For this review, take the finished solid that the model builds, in its own axes (mm). A direction names the side the tool comes from. Coordinates: 2 decimals unless noted, no trailing zeros. Loops run counter-clockwise (first coordinate to the right, second up) from the corner with the lowest first, then second, coordinate; pieces in that order, holes last. Notation, with made-up numbers: (-5.75, -34) - (45.25, -34) arc R6 cw to (45.25, -24) - close; hole circle Ø3 at (3, 54). An arc over 180 degrees is marked (long way). Answer as a JSON object with one key per item and string values. Group by question number.
Item 1: We need section A-A (y = 17.5). Give the boundary of the cut face in (x, z).
Item 2: Mouldability with a two-part tool opening along X and no side actions: class faces 4 (the flat face through (21, 2, -17)), 5 (the flat face through (0, 19, 4.3)) as released by +X, released by -X, zero draft, split by the parting line, or undercut.
Item 3: Clearance check with flat-ended pins moving along their axes: pin 1 (1.1 mm diameter, centred on x = 44, z = -35, fed in from +Y); pin 2 (1 mm diameter, centred on x = 33.5, y = 13, fed in from +Z); pin 3 (2 mm diameter, centred on x = -1.5, y = 7.5, fed in from -Z); pin 4 (4 mm diameter, centred on y = 13.5, z = -22, fed in from -X). State where each tip first meets the part, or that it passes through.
Item 4: We need section B-B (y = 9). Give the boundary of the cut face in (x, z), then the cut area to 3 significant figures.
Item 5: Tool access review of faces 1 (the flat face through (42.3, 19, 3)), 2 (the flat face through (45, 19, -15.2)), 3 (the flat face through (44.3, 10, -20)): name each direction out of +Z, -Z, +X, -X, +Y, -Y from which nothing blocks a thin tool from reaching the whole face with its end or side.
Item 6: To check wall thickness, follow line 1 (Z direction, x = 4.5, y = 4.25); line 2 (X direction, y = 12, z = -29); line 3 (Z direction, x = 1, y = 20.25). State the ranges of each line that lie inside material, in increasing order.
Item 7: We need section C-C (x = 34). Give the boundary of the cut face in (y, z), then the cut area to 3 significant figures.
Item 8: We need section D-D (z = -32.5). Give the boundary of the cut face in (x, y), then the cut area to 3 significant figures.
from build123d import *

# Parameters (mm, degrees)
SKETCH1_W           = 48.6
SKETCH1_H           = 37.6
SKETCH1_W_2         = 44.6
SKETCH1_H_2         = 33.6
SKETCH1_W_3         = 44
SKETCH1_H_3         = 33
BOSS_EXTRUDE1_DEPTH = 2
SKETCH1_3_W         = 48.6
SKETCH1_3_H         = 37.6
SKETCH1_3_W_2       = 44.6
SKETCH1_3_H_2       = 33.6
BOSS_EXTRUDE2_DEPTH = 22
SKETCH2_W           = 2
SKETCH2_H           = 16.6
CUT_EXTRUDE1_DEPTH  = 20
SKETCH3_W           = 2
SKETCH3_H           = 14
CUT_EXTRUDE2_DEPTH  = 11.5
FILLET1_R           = 5
SKETCH4_W           = 4
SKETCH4_H           = 2
BOSS_EXTRUDE3_DEPTH = 6
CHAMFER1_SIZE       = 2
SKETCH5_R           = 0.5
CUT_EXTRUDE4_DEPTH  = 6


with BuildPart() as part:
    # Sketch1 → Boss-Extrude1 (new body)
    # profile 1 of 3: a face of its own
    with BuildSketch(Plane(origin=(0, 0, 0), x_dir=(1, 0, 0), z_dir=(0, 1, 0))):
        with Locations((22, 16.5)):
            Rectangle(SKETCH1_W, SKETCH1_H)
        with Locations((22, 16.5)):
            Rectangle(SKETCH1_W_2, SKETCH1_H_2, mode=Mode.SUBTRACT)
    # profile 2 of 3: a face of its own
    with BuildSketch(Plane(origin=(0, 0, 0), x_dir=(1, 0, 0), z_dir=(0, 1, 0))):
        with Locations((22, 16.5)):
            Rectangle(SKETCH1_W_2, SKETCH1_H_2)
        with Locations((22, 16.5)):
            Rectangle(SKETCH1_W_3, SKETCH1_H_3, mode=Mode.SUBTRACT)
    # profile 3 of 3: a face of its own
    with BuildSketch(Plane(origin=(0, 0, 0), x_dir=(1, 0, 0), z_dir=(0, 1, 0))):
        with Locations((22, 16.5)):
            Rectangle(SKETCH1_W_3, SKETCH1_H_3)
    extrude(amount=BOSS_EXTRUDE1_DEPTH)

    # Sketch1<3> → Boss-Extrude2 (add)
    with BuildSketch(Plane(origin=(0, 0, 0), x_dir=(1, 0, 0), z_dir=(0, 1, 0))):
        with Locations((22, 16.5)):
            Rectangle(SKETCH1_3_W, SKETCH1_3_H)
        with Locations((22, 16.5)):
            Rectangle(SKETCH1_3_W_2, SKETCH1_3_H_2, mode=Mode.SUBTRACT)
    extrude(amount=BOSS_EXTRUDE2_DEPTH)

    # Sketch2 → Cut-Extrude1 (cut)
    with BuildSketch(Plane(origin=(0, 22, 0), x_dir=(1, 0, 0), z_dir=(0, 1, 0))):
        with Locations((-1.3, 16.5)):
            Rectangle(SKETCH2_W, SKETCH2_H)
    extrude(amount=-CUT_EXTRUDE1_DEPTH, mode=Mode.SUBTRACT)

    # Sketch3 → Cut-Extrude2 (cut)
    with BuildSketch(Plane(origin=(0, 22, 0), x_dir=(1, 0, 0), z_dir=(0, 1, 0))):
        with Locations((45.3, 8.2)):
            Rectangle(SKETCH3_W, SKETCH3_H)
    extrude(amount=-CUT_EXTRUDE2_DEPTH, mode=Mode.SUBTRACT)

    # Fillet1
    fillet1_edges = [part.edges().sort_by_distance(p)[0] for p in [
        (45.3, 10.5, -15.2),
        (45.3, 10.5, -1.2),
    ]]
    fillet(fillet1_edges, radius=FILLET1_R)

    # Sketch4 → Boss-Extrude3 (add)
    with BuildSketch(Plane(origin=(0, 22, 0), x_dir=(1, 0, 0), z_dir=(0, 1, 0))):
        with Locations((44.3, -3.3)):
            Rectangle(SKETCH4_W, SKETCH4_H)
        with Locations((-0.3, -3.3)):
            Rectangle(SKETCH4_W, SKETCH4_H)
        with Locations((-0.3, 36.3)):
            Rectangle(SKETCH4_W, SKETCH4_H)
        with Locations((44.3, 36.3)):
            Rectangle(SKETCH4_W, SKETCH4_H)
    extrude(amount=-BOSS_EXTRUDE3_DEPTH)

    # Chamfer1
    chamfer1_edges = [part.edges().sort_by_distance(p)[0] for p in [
        (-0.3, 16, 2.3),
        (44.3, 16, 2.3),
        (-0.3, 16, -35.3),
        (44.3, 16, -35.3),
    ]]
    chamfer(chamfer1_edges, length=CHAMFER1_SIZE - 0.0001)  # a hair under: the kernel refuses the full size

    # Sketch5 → Cut-Extrude4 (cut)
    with BuildSketch(Plane(origin=(0, 22, 0), x_dir=(1, 0, 0), z_dir=(0, 1, 0))):
        with Locations(Location((44.3, -2.3, 0), (0, 0, 270))):
            Circle(SKETCH5_R)
        with Locations(Location((-0.3, -2.3, 0), (0, 0, 270))):
            Circle(SKETCH5_R)
        with Locations(Location((-0.3, 35.3, 0), (0, 0, 270))):
            Circle(SKETCH5_R)
        with Locations(Location((44.3, 35.3, 0), (0, 0, 270))):
            Circle(SKETCH5_R)
    extrude(amount=-CUT_EXTRUDE4_DEPTH, mode=Mode.SUBTRACT)


solid = part.part
Check sheet entries:
{
 "1": {"outline": "(-2.3, -37.3) - (1.7, -37.3) - (1.7, -35.3) - (42.3, -35.3) - (42.3, -37.3) - (46.3, -37.3) - (46.3, -15.2) - (44.3, -15.2) - (44.3, -33.3) - (-0.3, -33.3) - (-0.3, -24.8) - (-2.3, -24.8) - close; (-2.3, -8.2) - (-0.3, -8.2) - (-0.3, 0.3) - (44.3, 0.3) - (44.3, -1.2) - (46.3, -1.2) - (46.3, 4.3) - (42.3, 4.3) - (42.3, 2.3) - (1.7, 2.3) - (1.7, 4.3) - (-2.3, 4.3) - close; hole circle Ø1 at (-0.3, -35.3); hole circle Ø1 at (-0.3, 2.3); hole circle Ø1 at (44.3, -35.3); hole circle Ø1 at (44.3, 2.3)"},
 "2": {"face 4": "undercut", "face 5": "zero draft"},
 "3": {"pin 1": "stops at y = 22", "pin 2": "stops at z = 2.3", "pin 3": "stops at z = -35.3", "pin 4": "stops at x = 44.3"},
 "4": {"outline": "(-2.3, -35.3) - (46.3, -35.3) - (46.3, 2.3) - (-2.3, 2.3) - (-2.3, -8.2) - (-0.3, -8.2) - (-0.3, 0.3) - (44.3, 0.3) - (44.3, -33.3) - (-0.3, -33.3) - (-0.3, -24.8) - (-2.3, -24.8) - close", "area": "296 mm2"},
 "5": {"face 1": "+Z, +Y, -Y", "face 2": "+X, -X, +Y", "face 3": "+Y"},
 "6": {"line 1": "z = -35.3 to -33.3, 0.3 to 2.3", "line 2": "x = -2.3 to -0.3, 44.3 to 46.3", "line 3": "z = -37.3 to -33.3, 0.3 to 4.3"},
 "7": {"outline": "(0, -35.3) - (22, -35.3) - (22, -33.3) - (2, -33.3) - (2, 0.3) - (22, 0.3) - (22, 2.3) - (0, 2.3) - close", "area": "155 mm2"},
 "8": {"outline": "(-2.3, 0) - (46.3, 0) - (46.3, 22) - (44.3, 22) - (44.3, 2) - (-0.3, 2) - (-0.3, 22) - (-2.3, 22) - close", "area": "177 mm2"}
}
